Design review of the part built by this model. Coordinates are the model's own, in mm. A direction names the side the tool comes from. Coordinates: 2 decimals unless noted, no trailing zeros. Loops run counter-clockwise (first coordinate to the right, second up) from the corner with the lowest first, then second, coordinate; pieces in that order, holes last. Notation, with made-up numbers: (85, -4.5) -> (132, -4.5) arc R9 cw to (132, 9.5) -> close; hole circle Ø8 at (17, 63.25). An arc over 180 degrees is marked (long way). Use one line per item in the form item = value. Start each with the question number.
1. Consider section B-B (x = 0). State the section outline as (y, z) points.
2. Consider section C-C (z = 2.1). State the section outline as (x, y) points, then the cut area to 3 significant figures.
3. Consider section D-D (x = 71). State the section outline as (y, z) points.
4. Machinability: for faces 5 (the face through (-42.47, 102.53, 1.97)), 6 (the face through (-39.8, 113.77, 2.03)), which of the approach directions +Z, -Z, +X, -X, +Y, -Y give a long, thin tool a straight path to every point of the face, cutting with its end or side? Answer none if there is none.
5. The part is to be moulded in two halves that separate along Y. For faces 1 (the face through (113.4, -39.7, 2)), 2 (the face through (-42.47, -102.53, 1.97)), 3 (the face through (142.45, 3.83, 1.97)), 4 (the face through (87, 2, 0)), say which applies: released by +Y, released by -Y, zero draft, split by the parting line, or undercut.
6. Consider section A-A (y = -11.5). State the section outline as (x, z) points, then the cut area to 3 significant figures.
7. For pin 1 (5 mm diameter, centred on x = 108, y = -65.5, fed in from -Z); pin 2 (2 mm diameter, centred on y = -59, z = 1.5, fed in from +X); pin 3 (1.5 mm diameter, centred on x = 14.5, z = 3, fed in from -Y), all flat-tipped, find the tip position at first contact; note any pin that passes through.
8. Wall thickness on line 1 (X direction, y = 1.5, z = 2.15); line 2 (Y direction, x = -5.5, z = 1.25); line 3 (Y direction, x = 19, z = 1.7): over which ranges is each line inside the solid? List them lowest first. Write a range as from..to.
Autodesk Inventor part; units mm, degrees
ref_plane "YZ Plane" through (0, 0, 0) normal (1, 0, 0) x (0, 1, 0)
ref_plane "XZ Plane" through (0, 0, 0) normal (0, 1, 0) x (-1, 0, 0)
ref_plane "XY Plane" through (0, 0, 0) normal (0, 0, 1) x (1, 0, 0)
sketch "Sketch2" plane through (0, 0, 0) normal (0, 0, 1) x (1, 0, 0)
  circle A0 centre (0, 0) radius 80.5
  circle A1 centre (0, 0) radius 142.5
  line L0 (0, 0) -> (-54.5324, 131.6528)
  line L1 (0, 0) -> (-54.5324, -131.6528)
  line L2 (0, 0) -> (-142.5, 0) construction
  point P0 (-30.806, -74.3723)
  point P1 (-30.806, 74.3723)
  dimension "d25" = 161
  dimension "d27" = 285
  dimension "d29" = 135
extrude "Plate2" add sketch "Sketch2" along normal blind 4 contours A0 L0 A1 L1 picked at (65.8732, 102.2302)
sketch "Sketch3" plane through (0, 0, 4) normal (0, 0, 1) x (1, 0, 0)
  circle A0 centre (0, 0) radius 120 construction
  arc A1 (31.0583, 115.9111) -> (-31.0583, 115.9111) centre (0, 0) ccw construction
  arc A2 (33.3877, 124.6044) -> (-33.3877, 124.6044) centre (0, 0) ccw
  arc A3 (28.7289, 107.2178) -> (-28.7289, 107.2178) centre (0, 0) ccw
  arc A4 (28.7289, 107.2178) -> (33.3877, 124.6044) centre (31.0583, 115.9111) ccw
  arc A5 (-33.3877, 124.6044) -> (-28.7289, 107.2178) centre (-31.0583, 115.9111) ccw
  line L0 (-31.0583, 115.9111) -> (0, 0)
  line L1 (0, 0) -> (31.0583, 115.9111)
  line L2 (0, 0) -> (0, 70.9879)
  dimension "d28" = 240
  dimension "d30" = 18
  dimension "d31" = 30
extrude "Cut1" cut sketch "Sketch3" against normal blind 4 contours A4 A3 A5 A2
pattern_circular "Circular Pattern1" count 4 over 360 about axis through (0, 0, 0) along (0, 0, 1) of "Cut1"
fillet "Corner Round1" radius 6 4 edges at (-54.5324, 131.6528, 2) (-30.806, 74.3723, 2) (-30.806, -74.3723, 2) (-54.5324, -131.6528, 2)
sketch "Sketch5" plane through (0, 0, 0) normal (0, 0, -1) x (-1, 0, 0)
  arc A0 (-107.2178, 28.7289) -> (-107.2178, -28.7289) centre (0, 0) ccw
  arc A1 (-124.6044, -33.3877) -> (-107.2178, -28.7289) centre (-115.9111, -31.0583) ccw
  arc A2 (-124.6044, 33.3877) -> (-124.6044, -33.3877) centre (0, 0) ccw
  arc A3 (-107.2178, 28.7289) -> (-124.6044, 33.3877) centre (-115.9111, 31.0583) ccw
  arc A4 (-28.7289, -107.2178) -> (28.7289, -107.2178) centre (0, 0) ccw
  arc A5 (33.3877, -124.6044) -> (28.7289, -107.2178) centre (31.0583, -115.9111) ccw
  arc A6 (-33.3877, -124.6044) -> (33.3877, -124.6044) centre (0, 0) ccw
  arc A7 (-28.7289, -107.2178) -> (-33.3877, -124.6044) centre (-31.0583, -115.9111) ccw
  arc A8 (28.7289, 107.2178) -> (-28.7289, 107.2178) centre (0, 0) ccw
  arc A9 (-33.3877, 124.6044) -> (-28.7289, 107.2178) centre (-31.0583, 115.9111) ccw
  arc A10 (33.3877, 124.6044) -> (-33.3877, 124.6044) centre (0, 0) ccw
  arc A11 (28.7289, 107.2178) -> (33.3877, 124.6044) centre (31.0583, 115.9111) ccw
  arc A12 (48.6927, -133.9226) -> (52.1858, -125.9877) centre (46.6425, -128.2838) ccw
  line L0 (33.0224, -79.7231) -> (52.1858, -125.9877)
  arc A13 (33.0224, -79.7231) -> (25.573, -76.33) centre (27.4791, -82.0192) ccw
  arc A14 (25.573, 76.33) -> (25.573, -76.33) centre (0, 0) ccw
  arc A15 (25.573, 76.33) -> (33.0224, 79.7231) centre (27.4791, 82.0192) ccw
  line L1 (52.1858, 125.9877) -> (33.0224, 79.7231)
  arc A16 (52.1858, 125.9877) -> (48.6927, 133.9226) centre (46.6425, 128.2838) ccw
  arc A17 (48.6927, 133.9226) -> (48.6927, -133.9226) centre (0, 0) ccw
  line L2 (14.6903, 87.3165) -> (-84.3637, 63.9504)
  line L3 (-84.3637, 63.9504) -> (-84.3637, -55.2862)
  line L4 (-84.3637, -55.2862) -> (17.3285, -91.5935)
equation "\"d17\" = Thickness"
equation "\"d14\" = Thickness"
equation "\"BendReliefWidth\" = Thickness"
equation "\"BendReliefDepth\" = 0.5 * Thickness"
equation "\"CornerReliefSize\" = 4 * Thickness"
equation "\"MinimumRemnant\" = 2 * Thickness"
equation "\"TransitionRadius\" = BendRadius"
equation "\"JacobiRadiusSize\" = BendRadius"
equation "\"GapSize\" = Thickness"
properties part number "PNS 1707 funnel flange" material "Steel"
Geometry check:
q1.outline = (-142.5, 0) -> (-129, 0) -> (-129, 4) -> (-142.5, 4) -> close; (-111, 0) -> (-80.5, 0) -> (-80.5, 4) -> (-111, 4) -> close; (80.5, 0) -> (111, 0) -> (111, 4) -> (80.5, 4) -> close; (129, 0) -> (142.5, 0) -> (142.5, 4) -> (129, 4) -> close
q2.outline = (-52.19, -125.99) arc R6 ccw to (-48.69, -133.92) arc R142.5 ccw (long way) to (-48.69, 133.92) arc R6 ccw to (-52.19, 125.99) -> (-33.02, 79.72) arc R6 ccw to (-25.57, 76.33) arc R80.5 cw (long way) to (-25.57, -76.33) arc R6 ccw to (-33.02, -79.72) -> close; hole (-33.39, -124.6) arc R129 ccw to (33.39, -124.6) arc R9 ccw to (28.73, -107.22) arc R111 cw to (-28.73, -107.22) arc R9 ccw to start; hole (-33.39, 124.6) arc R9 ccw to (-28.73, 107.22) arc R111 cw to (28.73, 107.22) arc R9 ccw to (33.39, 124.6) arc R129 ccw to start; hole (107.22, -28.73) arc R9 ccw to (124.6, -33.39) arc R129 ccw to (124.6, 33.39) arc R9 ccw to (107.22, 28.73) arc R111 cw to start
q2.area = 23,000 mm²
q3.outline = (-123.55, 0) -> (-37.94, 0) -> (-37.94, 4) -> (-123.55, 4) -> close; (37.94, 0) -> (123.55, 0) -> (123.55, 4) -> (37.94, 4) -> close
q4.face_5 = +Z, -Z, -X
q4.face_6 = +Z, -Z
q5.face_1 = undercut
q5.face_2 = undercut
q5.face_3 = split by the parting line
q5.face_4 = zero draft
q6.outline = (79.67, 0) -> (110.4, 0) -> (110.4, 4) -> (79.67, 4) -> close; (128.49, 0) -> (142.04, 0) -> (142.04, 4) -> (128.49, 4) -> close
q6.area = 177 mm²
q7.pin_1 = 0
q7.pin_2 = 130.16
q7.pin_3 = -141.84
q8.line_1 = 80.49..110.99, 128.99..142.49
q8.line_2 = -142.39..-128.88, -110.86..-80.31, 80.31..110.86, 128.88..142.39
q8.line_3 = -141.23..-127.59, -109.36..-78.23, 78.23..109.36, 127.59..141.23
